Part model, mm, in its own coordinate system. Round coordinates to 2 decimals unless told otherwise and drop trailing zeros. Loops run counter-clockwise (first coordinate to the right, second up) from the corner with the lowest first, then second, coordinate; pieces in that order, holes last.
1) Band-saw the part on A-A, the plane x = 47. Write the cut outline in (y, z).
2) Drop a flat-ended pin along its axis: P1, Ø5, axis at y = 7, z = 11, coming from the -X side. Give the stop position or say it passes through.
3) Band-saw the part on B-B, the plane z = 9.75. Write the cut outline in (x, y).
4) Probe line 1 (X direction, y = 6, z = 12.4); line 2 (Z direction, x = 216.5, y = 5); line 3 (Y direction, x = 14, z = -1.05). List the from-to ranges inside material, lowest first.
5) Band-saw the part on C-C, the plane x = 165. Write the cut outline in (y, z), then the cut area to 3 significant figures.
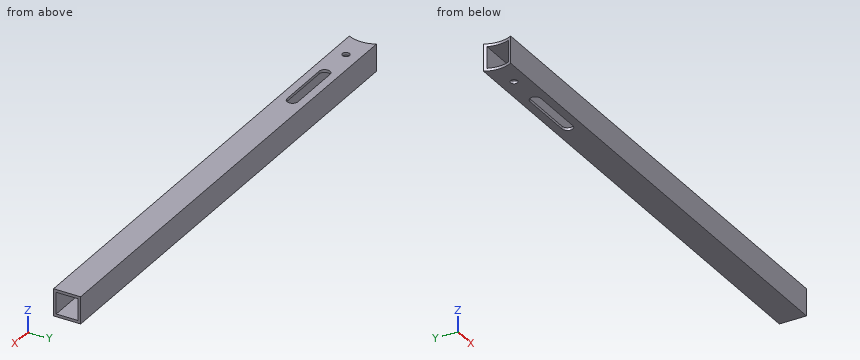
Autodesk Inventor part; units mm, degrees
ref_plane "YZ Plane" through (0, 0, 0) normal (1, 0, 0) x (0, 1, 0)
ref_plane "XZ Plane" through (0, 0, 0) normal (0, 1, 0) x (-1, 0, 0)
ref_plane "XY Plane" through (0, 0, 0) normal (0, 0, 1) x (1, 0, 0)
sketch "Sketch1" plane through (0, 0, 0) normal (1, 0, 0) x (0, 1, 0)
  line L0 (0, 0) -> (12, 0)
  line L1 (12, 0) -> (12, 12)
  line L2 (12, 12) -> (0, 12)
  line L3 (0, 12) -> (0, 0)
  line L4 (-1.5, 13.5) -> (13.5, 13.5)
  line L5 (13.5, 13.5) -> (13.5, -1.5)
  line L6 (13.5, -1.5) -> (-1.5, -1.5)
  line L7 (-1.5, -1.5) -> (-1.5, 13.5)
  dimension "FalVastagsag" = 1.5
  dimension "BelsoAtmero" = 12
  dimension "d2" = 12
extrude "Extrusion1" add sketch "Sketch1" along normal blind 275 and the other way blind 15
sketch "Sketch2" plane through (0, -1.5, 13.5) normal (0, 0, 1) x (1, 0, 0)
  line L0 (0, 0) -> (0, 15)
  line L1 (0, 0) -> (275, 0)
  circle A0 centre (-16, 7.5) radius 16
  circle A1 centre (-16, 7.5) radius 30
  circle A2 centre (14, 7.5) radius 2
  point P0 (0, 1.5)
  dimension "d22" = 60
  dimension "d8" = 32
  dimension "d9" = 16
  dimension "d23" = 4
sketch "Sketch4" plane through (0, 0, 0) normal (-1, 0, 0) x (0, 0, 1)
  line L0 (0, 0) -> (12, 0)
  line L1 (12, 0) -> (12, 12)
  line L2 (12, 12) -> (0, 12)
  line L3 (0, 12) -> (0, 0)
  line L4 (-1.5, -1.5) -> (13.5, -1.5)
  line L5 (13.5, -1.5) -> (13.5, 13.5)
  line L6 (13.5, 13.5) -> (-1.5, 13.5)
  line L7 (-1.5, 13.5) -> (-1.5, -1.5)
extrude "Extrusion2" add sketch "Sketch4" along normal blind 10
extrude "Extrusion3" cut sketch "Sketch2" against normal through all contours A0
sketch "Sketch5" plane through (-16, 6, 13.5) normal (0, 0, 1) x (1, 0, 0)
  arc A0 (50, 2.9901) -> (50, -3.0099) centre (50, -0.0099) ccw
  arc A1 (80, -3.0099) -> (80, 2.9901) centre (80, -0.0099) ccw
  line L0 (50, 2.9901) -> (80, 2.9901)
  line L1 (80, -3.0099) -> (50, -3.0099)
  arc A2 (14.1333, -7.5) -> (14.1333, 7.5) centre (0, 0) ccw
  point P0 (16, -6)
  dimension "d16" = 6
  dimension "d17" = 6
  dimension "d18" = 30
  dimension "d19" = 50
extrude "Extrusion4" cut sketch "Sketch5" against normal through all
extrude "Extrusion5" cut sketch "Sketch2" against normal through all contours A2 A1 | A1 A2 picked at (14.5954, 6.9828) picked at (13.3724, 7.0462)
mirror "Mirror2" [suppressed]
equation "\"FalVastagsag\" = ZártSzelvényFalVastagság"
equation "\"BelsoAtmero\" = ZártSzelvényBelsőÁtmérő"
equation "\"d2\" = ZártSzelvényBelsőÁtmérő"
equation "\"d22\" = 2 * PorvedoRogzitesJatekSugara"
equation "\"d8\" = CsapágyHázKülsőÁtmérő"
equation "\"d9\" = 0.5 * CsapágyHázKülsőÁtmérő"
equation "\"ZártSzelvényFalVastagság\" = 1.5"
equation "\"ZártSzelvényBelsőÁtmérő\" = 12"
equation "\"CsapágyHázKülsőÁtmérő\" = 32"
equation "\"ZártSzelvényKülsőÁtmérő\" = 15"
equation "\"CsapágyBelsőÁtmérő\" = 12"
equation "\"CsapágyKülsőÁtmérő\" = 28"
equation "\"CsapágyHázBelsőÁtmérő\" = 26"
equation "\"CTipHoszza\" = 400"
equation "\"ATipHoszza\" = 400"
equation "\"BTipHoszza\" = 70"
equation "\"CsapágyHázHoszza\" = 45"
equation "\"CsapágySzélesége\" = 8"
properties part number "KétvégenMartSzelvény" material "Acetal Resin, Black"
Reported:
1. outline: (-1.5, -1.5) - (2.99, -1.5) - (2.99, 0) - (0, 0) - (0, 12) - (2.99, 12) - (2.99, 13.5) - (-1.5, 13.5) - close; (8.99, -1.5) - (13.5, -1.5) - (13.5, 13.5) - (8.99, 13.5) - (8.99, 12) - (12, 12) - (12, 0) - (8.99, 0) - close
2. P1: stops at x = -0.34
3. outline: (-1.87, -1.5) - (275, -1.5) - (275, 0) - (-1.17, 0) arc R16 cw to start; (-1.87, 13.5) arc R16 cw to (-1.17, 12) - (275, 12) - (275, 13.5) - close
4. line 1: x = 0 to 12, 16 to 31, 67 to 275
4. line 2: z = -1.5 to 0, 12 to 13.5
4. line 3: y = -1.5 to 4, 8 to 13.5
5. outline: (-1.5, -1.5) - (13.5, -1.5) - (13.5, 13.5) - (-1.5, 13.5) - close; hole (0, 0) - (12, 0) - (12, 12) - (0, 12) - close
5. area: 81.0 mm2
